Model file for the job. Use its own axes, mm. Coordinates: 2 decimals unless noted, no trailing zeros. Order: outer loops, then holes, each group sorted by start corner. A loop starts at its lowest first (then second) coordinate and runs counter-clockwise, first axis right, second up. Notation, with made-up numbers: (-28, 56) - (13, 56) arc R12 cw to (13, 66) - close; hole circle Ø10 at (44.5, -38.5). An arc over 180 degrees is marked (long way). Put each result on its own line as item: value. Start each with the question number.
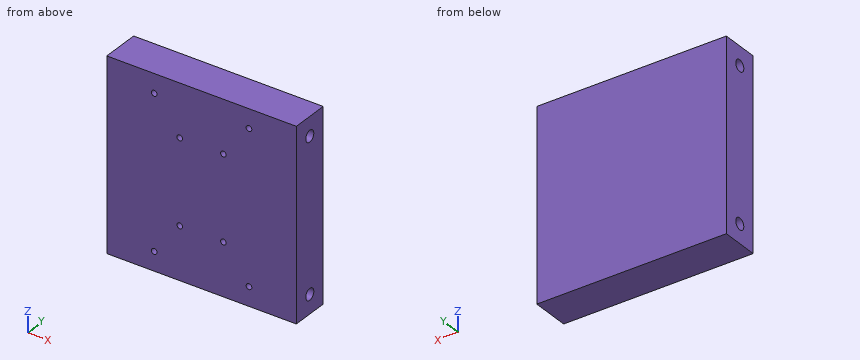
Autodesk Fusion 360 part; units mm, degrees
sketch "Esquisse1" plane through (0, 0, 0) normal (0, 1, 0) x (1, 0, 0)
  line L0 (0, 0) -> (100, 0)
  line L1 (100, 0) -> (100, 100)
  line L2 (100, 100) -> (0, 100)
  line L3 (0, 100) -> (0, 0)
  dimension "d1" = 100
  dimension "d2" = 100
extrude "Extrusion1" add sketch "Esquisse1" along normal blind 20
sketch "Esquisse2" plane through (100, 0, 0) normal (1, 0, 0) x (0, 0, -1)
  line L0 (0, 0) -> (100, 0)
  line L1 (100, 0) -> (100, 20)
  line L2 (100, 20) -> (0, 20)
  line L3 (0, 20) -> (0, 0)
  line L4 (0, 10) -> (37, 10)
  circle A0 centre (10, 10) radius 3
  line L5 (50, 20) -> (50, 0)
  circle A1 centre (90, 10) radius 3
  dimension "d5" = 6
  dimension "d6" = 10
extrude "Extrusion2" cut sketch "Esquisse2" against normal blind 10 contours L4 A0 | L4 A0 | A1
sketch "Esquisse3" plane through (0, 0, 0) normal (-1, 0, 0) x (0, 0, 1)
  line L0 (-100, 0) -> (0, 0)
  line L1 (0, 0) -> (0, 20)
  line L2 (0, 20) -> (-100, 20)
  line L3 (-100, 20) -> (-100, 0)
  line L4 (-100, 10) -> (-70, 10)
  line L5 (-50, 20) -> (-50, 0)
  circle A0 centre (-90, 10) radius 3
  circle A1 centre (-10, 10) radius 3
  dimension "d9" = 6
  dimension "d10" = 10
extrude "Extrusion3" cut sketch "Esquisse3" against normal blind 10 contours L4 A0 | L4 A0 | A1
sketch "Esquisse4" plane through (0, 0, 0) normal (0, -1, 0) x (1, 0, 0)
  line L0 (0, 0) -> (0, -100)
  line L1 (0, -100) -> (100, -100)
  line L2 (100, -100) -> (100, 0)
  line L3 (100, 0) -> (0, 0)
  line L4 (0, -5) -> (20, -5)
  line L5 (20, -5) -> (20, 0)
  line L6 (80, 0) -> (80, -5)
  line L7 (80, -5) -> (100, -5)
  line L8 (0, -95) -> (20, -95)
  line L9 (20, -95) -> (20, -100)
  line L10 (80, -100) -> (80, -95)
  line L11 (80, -95) -> (100, -95)
  line L12 (20, -5) -> (80, -5)
  line L13 (80, -95) -> (20, -95)
  line L14 (20, -95) -> (20, -5)
  line L15 (80, -5) -> (80, -95)
  line L16 (20, -90) -> (25, -90)
  line L17 (25, -90) -> (25, -95)
  line L18 (80, -90) -> (75, -90)
  line L19 (75, -90) -> (75, -95)
  circle A0 centre (25, -90) radius 1.5
  circle A1 centre (75, -90) radius 1.5
  line L20 (20, -10) -> (25, -10)
  line L21 (25, -10) -> (25, -5)
  line L22 (75, -5) -> (75, -10)
  line L23 (75, -10) -> (80, -10)
  circle A2 centre (25, -10) radius 1.5
  circle A3 centre (75, -10) radius 1.5
  line L24 (35.75, -100) -> (35.75, -75)
  line L25 (35.75, -75) -> (0, -75)
  line L26 (35.75, 0) -> (35.75, -25)
  line L27 (35.75, -25) -> (0, -25)
  line L28 (64.25, 0) -> (64.25, -25)
  line L29 (64.25, -25) -> (100, -25)
  line L30 (100, -75) -> (64.25, -75)
  line L31 (64.25, -75) -> (64.25, -100)
  line L32 (64.25, -75) -> (35.75, -75)
  line L33 (35.75, -75) -> (35.75, -25)
  line L34 (35.75, -25) -> (64.25, -25)
  line L35 (64.25, -25) -> (64.25, -75)
  line L36 (61.5, -75) -> (61.5, -72.25)
  line L37 (61.5, -72.25) -> (64.25, -72.25)
  line L38 (38.5, -75) -> (38.5, -72.25)
  line L39 (38.5, -72.25) -> (35.75, -72.25)
  line L40 (38.5, -25) -> (38.5, -27.75)
  line L41 (38.5, -27.75) -> (35.75, -27.75)
  line L42 (61.5, -25) -> (61.5, -27.75)
  line L43 (61.5, -27.75) -> (64.25, -27.75)
  circle A4 centre (38.5, -72.25) radius 1.5
  circle A5 centre (61.5, -72.25) radius 1.5
  circle A6 centre (38.5, -27.75) radius 1.5
  circle A7 centre (61.5, -27.75) radius 1.5
  dimension "d13" = 5
  dimension "d14" = 20
  dimension "d15" = 5
  dimension "d16" = 20
  dimension "d17" = 20
  dimension "d18" = 20
  dimension "d19" = 5
  dimension "d20" = 5
  dimension "d21" = 5
  dimension "d22" = 5
  dimension "d23" = 5
  dimension "d24" = 5
  dimension "d25" = 3
  dimension "d26" = 3
  dimension "d27" = 5
  dimension "d28" = 5
  dimension "d29" = 5
  dimension "d30" = 5
  dimension "d31" = 3
  dimension "d32" = 3
  dimension "d35" = 25
  dimension "d36" = 25
  dimension "d37" = 35.75
  dimension "d38" = 35.75
  dimension "d39" = 25
  dimension "d40" = 25
  dimension "d41" = 35.75
  dimension "d42" = 35.75
  dimension "d43" = 2.75
  dimension "d44" = 2.75
  dimension "d45" = 2.75
  dimension "d46" = 2.75
  dimension "d47" = 2.75
  dimension "d48" = 2.75
  dimension "d49" = 2.75
  dimension "d50" = 2.75
  dimension "d51" = 3
  dimension "d52" = 3
  dimension "d53" = 3
  dimension "d54" = 3
extrude "Extrusion4" cut sketch "Esquisse4" against normal blind 10 contours L20 L21 A2 | L20 L21 A2 | L16 L17 A0 | L16 L17 A0 | L22 L23 A3 | L22 L23 A3 | L18 L19 A1 | L18 L19 A1
extrude "Extrusion5" cut sketch "Esquisse4" against normal blind 10 contours L40 L41 A6 | L40 L41 A6 | L38 L39 A4 | L38 L39 A4 | L42 L43 A7 | L42 L43 A7 | L36 L37 A5 | L36 L37 A5
Item 1: Slice it at A-A, the plane z = -10. Give the cut face in (x, y), plus the area to 3 significant figures.
Item 2: Slice it at D-D, the plane z = -27.75. Give the cut face in (x, y).
Item 3: Wall check: line 1 along Z through (x, y) = (61.5, 2.5); line 2 along X through (y, z) = (6.25, -90); line 3 along Z through (x, y) = (75, 2.5). Give the ranges that are in metal, low to high.
Item 4: Slice it at B-B, the plane x = 61.5. Give the cut face in (y, z).
Item 5: Slice it at C-C, the plane y = 11.5. Give the cut face in (x, z), plus the area to 3 significant figures.
Item 6: Flat gauge pins, fed straight in: pin 1 Ø1.5 at (x, z) = (24.5, -90) entering from -Y; pin 2 Ø4 at (y, z) = (13, -76) entering from -X; pin 3 Ø3.5 at (y, z) = (10, -90) entering from +X; pin 4 Ø5 at (y, z) = (10, -10) entering from -X. Where does each tip first touch, or does it go through?
Here are the results:
1. outline: (0, 0) - (23.5, 0) - (23.5, 10) - (26.5, 10) - (26.5, 0) - (73.5, 0) - (73.5, 10) - (76.5, 10) - (76.5, 0) - (100, 0) - (100, 7) - (90, 7) - (90, 13) - (100, 13) - (100, 20) - (0, 20) - (0, 13) - (10, 13) - (10, 7) - (0, 7) - close
1. area: 1,820 mm^2
2. outline: (0, 0) - (37, 0) - (37, 10) - (40, 10) - (40, 0) - (60, 0) - (60, 10) - (63, 10) - (63, 0) - (100, 0) - (100, 20) - (0, 20) - close
3. line 1: z = -100 to -73.75, -70.75 to -29.25, -26.25 to 0
3. line 2: x = 0 to 23.5, 26.5 to 73.5, 76.5 to 100
3. line 3: z = -100 to -91.5, -88.5 to -11.5, -8.5 to 0
4. outline: (0, -100) - (20, -100) - (20, 0) - (0, 0) - (0, -26.25) - (10, -26.25) - (10, -29.25) - (0, -29.25) - (0, -70.75) - (10, -70.75) - (10, -73.75) - (0, -73.75) - close
5. outline: (0, -100) - (100, -100) - (100, -92.6) - (90, -92.6) - (90, -87.4) - (100, -87.4) - (100, -12.6) - (90, -12.6) - (90, -7.4) - (100, -7.4) - (100, 0) - (0, 0) - (0, -7.4) - (10, -7.4) - (10, -12.6) - (0, -12.6) - (0, -87.4) - (10, -87.4) - (10, -92.6) - (0, -92.6) - close
5. area: 9,790 mm^2
6. pin 1: stops at y = 10
6. pin 2: stops at x = 0
6. pin 3: stops at x = 90
6. pin 4: stops at x = 10
